Check sheet for the modelled part. Datum: model origin and axes. Units: mm. A direction names the side the tool comes from. Round coordinates to 2 decimals unless told otherwise and drop trailing zeros. Order: outer loops, then holes, each group sorted by start corner. A loop starts at its lowest first (then second) coordinate and runs counter-clockwise, first axis right, second up. Notation, with made-up numbers: M 40.5,54 L 93.5,54 A23 ccw 93.5,67 Z; hole C 52,-31.5 d2. An arc over 180 degrees is marked long. One line per item, written item: value. Start each with the question number.
(1) Cross-section at A-A, the plane y = 3. Enter the section's corners in (x, z), and give its area (3 significant figures).
(2) Depth check by flat-ended pin: pin 1 Ø5 at (y, z) = (6.5, 8.5) entering from +X; pin 2 Ø6 at (x, z) = (-9.5, 6.5) entering from -Y (3 decimals); pin 3 Ø3 at (y, z) = (6.5, 13.5) entering from -X; pin 4 Ø1.5 at (x, z) = (3.5, 13.5) entering from -Y. Enter the tip coordinate at first touch or a pass-through.
(3) Thickness scan on L1, parallel to X at y = 7.75, z = 18.25; L2, parallel to Y at x = 3, z = 18.25; L3, parallel to Y at x = -13.5, z = 12.75 (3 decimals). Record the ranges inside material, lowest first.
(4) Access from +Z, -Z, +X, -X, +Y, -Y to the whole of each face (thin tool, end or side, straight path). Record for faces 1 (the face through (0, 5, 10)), 2 (the face through (-22.225, 11, 10)), 3 (the face through (7.938, 5, 10)).
from build123d import *

# Parameters (mm, degrees)
F1_DEPTH = 20


with BuildPart() as f1:
    # F0 (on Top) → F1 (new body)
    with BuildSketch(Plane.XY):
        with BuildLine():
            Line((0, 9.525), (0, 0))
            Line((0, 0), (7.9375, 0))
            Line((7.9375, 0), (7.9375, 9.525))
            Line((7.9375, 9.525), (30.1625, 9.525))
            Line((30.1625, 9.525), (30.1625, 11.525))
            add(Edge.make_bspline(
                [(-22.225, 11.525), (-16.82, 15.041926), (3.968839, 16.008074), (24.757321, 15.041926), (30.1625, 11.525)],
                knots=[0, 0, 0, 0, 26.497406, 52.994813, 52.994813, 52.994813, 52.994813], degree=3))
            Line((-22.225, 11.525), (-22.225, 9.525))
            Line((-22.225, 9.525), (0, 9.525))
        make_face()
    extrude(amount=F1_DEPTH)


solid = f1.part
Values found:
1. outline: M 0,0 L 7.94,0 L 7.94,20 L 0,20 Z
1. area: 159 mm^2
2. pin 1: x = 7.94
2. pin 2: y = 9.525
2. pin 3: x = 0
2. pin 4: y = 0
3. L1: 0 to 7.94
3. L2: 0 to 15.52
3. L3: 9.525 to 14.48
4. face 1: +Z, -Z, -X, -Y
4. face 2: +Z, -Z, -X, +Y, -Y
4. face 3: +Z, -Z, +X, -Y
